Geometry: final body of the model. Coordinates: model frame, mm. Face numbers are marked on the shaded views. A direction names the side the tool comes from. Coordinates: 2 decimals unless noted, no trailing zeros. Write each loop counter-clockwise with the first axis right and the second up, starting at its lowest first coordinate (ties: lowest second). Pieces come first, ordered by that corner, then holes. Notation, with made-up numbers: (51, -5.75) -> (106, -5.75) arc R31 ccw to (106, 28.25) -> close; hole circle Ø1 at (9.5, 82.25). An arc over 180 degrees is marked (long way). One line per item, written item: value.
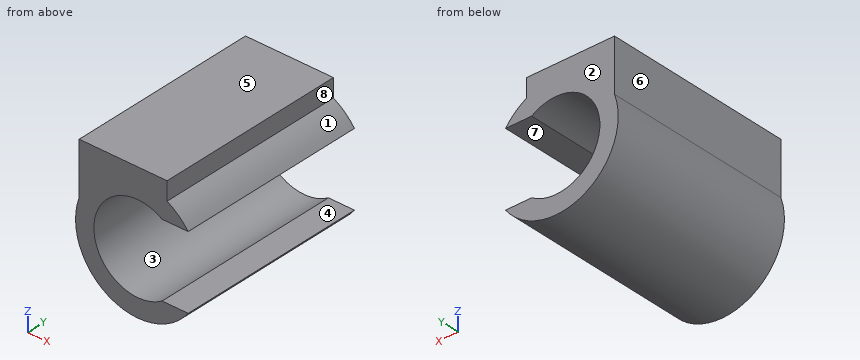
```python
from build123d import *

# Parameters (mm, degrees)
F1_DEPTH  = 73.66
F3_DEPTH  = 73.66
F4_W      = 25.4
F4_H      = 6.349999
F4_H_2    = 6.35
F5_DEPTH  = 69.85
F6_W      = 12.7
F6_H      = 63.5
F7_DEPTH  = 63.5
F8_W      = 25.4
F8_H      = 82.55
F9_DEPTH  = 57.15
F10_W     = 25.4
F10_H     = 6.349999
F11_DEPTH = 69.851


with BuildPart() as f1:
    # F0 (on Front) → F1 (new body)
    with BuildSketch(Plane.XZ):
        with BuildLine():
            ThreePointArc((2.106057, -3.175), (-3.81, 0), (2.106057, 3.175))
            Line((2.106057, 3.175), (4.364903, 3.175))
            ThreePointArc((4.364903, 3.175), (-5.3975, 0), (4.364903, -3.175))
            Line((4.364903, -3.175), (2.106057, -3.175))
        make_face()
    extrude(amount=F1_DEPTH)

    # F2 (on face) → F3 (join, through all)
    with BuildSketch(Plane.XZ.offset(73.66)):
        with BuildLine():
            Line((-5.08, 6.35), (-5.08, 1.823899))
            ThreePointArc((-5.08, 1.823899), (-1.942098, 5.035997), (2.54, 4.7625))
            Line((2.54, 4.7625), (2.54, 6.35))
            Line((2.54, 6.35), (-5.08, 6.35))
        make_face()
    extrude(amount=-F3_DEPTH)

    # F4 (on face) → F5 (join)
    with BuildSketch(Plane.XY.offset(6.35)):
        with Locations((-1.27, -65.405)):
            Rectangle(F4_W, F4_H)
        with Locations((-1.27, -8.255)):
            Rectangle(F4_W, F4_H_2)
    extrude(amount=F5_DEPTH)

    # F6 (on face) → F7 (cut, through all)
    with BuildSketch(Plane.XZ.offset(68.58)):
        with Locations((-1.27, 44.45)):
            Rectangle(F6_W, F6_H)
    extrude(amount=-F7_DEPTH, mode=Mode.SUBTRACT)

    # F8 (on face) → F9 (cut)
    with BuildSketch(Plane(origin=(0, 0, 0), x_dir=(-1, 0, 0), z_dir=(0, 1, 0))):
        with Locations((1.27, 34.925)):
            Rectangle(F8_W, F8_H)
    extrude(amount=-F9_DEPTH, mode=Mode.SUBTRACT)

    # F10 (on face) → F11 (cut, through all)
    with BuildSketch(Plane(origin=(0, 0, 6.35), x_dir=(1, 0, 0), z_dir=(0, 0, -1))):
        with Locations((-1.27, 65.405)):
            Rectangle(F10_W, F10_H)
    extrude(amount=-F11_DEPTH, mode=Mode.SUBTRACT)


solid = f1.part
```
(1) Line query: line 1 (Z direction, x = 0, y = -67); line 2 (X direction, y = -65.5, z = 0); line 3 (X direction, y = -68.5, z = 5). Output: solid intervals per line, ascending. Write a range as [from, to].
Responses:
line 1: z = [-5.4, -3.81], [3.81, 6.35]
line 2: x = [-5.4, -3.81]
line 3: x = [-5.08, 2.54]
(2) Pull-direction query (Z, two-part tool) for the marked faces 1, 2, 3 and 4; classes: released by +Z, released by -Z, zero draft, split by the parting line, or undercut.
Responses:
face 1: released by +Z
face 2: zero draft
face 3: undercut
face 4: undercut
(3) Section D-D (z = 1). Return the cut outline in (x, y).
Responses:
outline: (-5.3, -73.66) -> (-3.68, -73.66) -> (-3.68, -57.15) -> (-5.3, -57.15) -> close
(4) First-contact query: pin 1 (0.8 mm diameter, centred on y = -67, z = 5, fed in from +X); pin 2 (1.8 mm diameter, centred on x = 2.5, y = -62.5, fed in from -Z); pin 3 (1.4 mm diameter, centred on y = -63.5, z = 3, fed in from -X). Flat tips, straight axial feed; report the tip coordinate or a pass-through.
Responses:
pin 1: stops at x = 2.82
pin 2: stops at z = -5.15
pin 3: stops at x = -5.08
(5) Section C-C (x = 1). Return the cut outline in (y, z), then the cut area to 3 significant figures.
Responses:
outline: (-73.66, -5.3) -> (-57.15, -5.3) -> (-57.15, -3.68) -> (-73.66, -3.68) -> close; (-73.66, 3.68) -> (-57.15, 3.68) -> (-57.15, 6.35) -> (-73.66, 6.35) -> close
area: 71.0 mm2
(6) Reachability of the marked faces 5, 6, 7 and 8 from +Z, -Z, +X, -X, +Y, -Y: full face, straight path, thin tool, end or side. Return the list, or none.
Responses:
face 5: +Z, +X, -X, +Y, -Y
face 6: +Z, -X, +Y, -Y
face 7: +X, +Y, -Y
face 8: +Z, +X, +Y, -Y
(7) Section A-A (x = 0). Return the cut outline in (y, z), then the cut area to 3 significant figures.
Responses:
outline: (-73.66, -5.4) -> (-57.15, -5.4) -> (-57.15, -3.81) -> (-73.66, -3.81) -> close; (-73.66, 3.81) -> (-57.15, 3.81) -> (-57.15, 6.35) -> (-73.66, 6.35) -> close
area: 68.1 mm2
